from build123d import *

# Parameters (mm, degrees)
ESQUISSE1_R                  = 32.75
ESQUISSE1_R_2                = 30.75
BOSS_EXTRU_1_DEPTH           = 25
ESQUISSE2_W                  = 30
ESQUISSE2_H                  = 4
ENL_V_MAT_EXTRU_1_DEPTH      = 53.631976972
R_P_TITION_CIRCULAIRE1_COUNT = 4


with BuildPart() as part:
    # Esquisse1 → Boss.-Extru.1 (new body)
    with BuildSketch(Plane(origin=(0, 0, 0), x_dir=(1, 0, 0), z_dir=(0, 1, 0))):
        with Locations(Location((0, 0, 0), (0, 0, 270))):
            Circle(ESQUISSE1_R)
        with Locations(Location((0, 0, 0), (0, 0, 270))):
            Circle(ESQUISSE1_R_2, mode=Mode.SUBTRACT)
    extrude(amount=BOSS_EXTRU_1_DEPTH)

    # Esquisse2 → Enlèv. mat.-Extru.1 (cut, through all)
    with BuildSketch(Plane.XY):
        with Locations((0, 17)):
            Rectangle(ESQUISSE2_W, ESQUISSE2_H)
    enl_v_mat_extru_1 = extrude(amount=-ENL_V_MAT_EXTRU_1_DEPTH, mode=Mode.SUBTRACT)

    # Répétition circulaire1: Enlèv. mat.-Extru.1 ×4 about axis
    r_p_tition_circulaire1_axis = Axis((0, 0, 0), (0, 1, 0))
    for i in range(1, R_P_TITION_CIRCULAIRE1_COUNT):
        add(enl_v_mat_extru_1.rotate(r_p_tition_circulaire1_axis, i * 360 / R_P_TITION_CIRCULAIRE1_COUNT), mode=Mode.SUBTRACT)


solid = part.part
Geometry: final body of the model. Coordinates: model frame, mm. A direction names the side the tool comes from. Give positions to 0.01 mm unless a question says otherwise; leave off trailing zeros. Loops run counter-clockwise (first coordinate to the right, second up) from the corner with the lowest first, then second, coordinate; pieces in that order, holes last. Notation, with made-up numbers: M 45,89.25 L 95,89.25 A31 ccw 95,128.25 Z; hole C 3.25,-3.5 d1. An arc over 180 degrees is marked long. Put each result on its own line as item: value. Start each with the question number.
1) Cut plane A-A (z = 0). Output: boundary loops of the cut face in (x, y).
2) Contact query for flat-ended pins moving along their axis: pin 1 (6 mm diameter, centred on y = 7, z = 10, fed in from +X); pin 2 (1.8 mm diameter, centred on x = -28, y = 17.5, fed in from +Z); pin 3 (1.8 mm diameter, centred on y = 18, z = 28.5, fed in from -X). Output: stop coordinate, or through.
3) Cut plane B-B (x = 0). Output: boundary loops of the cut face in (y, z), then the cut area to 3 significant figures.
4) Ray query, line 1 along X through (y, z) = (19.75, 0); line 2 along Y through (x, z) = (29, 14.5); line 3 along X through (y, z) = (8.75, -15). Return the intervals inside material, ascending.
5) Cut plane C-C (y = 11.5). Output: boundary loops of the cut face in (x, z), then the cut area to 3 significant figures.
6) Pull-direction query (X, two-part tool) for faces 1 (the flat face through (31, 15, 0)), 2 (the flat face through (-15, 17, 28)); classes: pulls with the +X half, pulls with the -X half, needs draft (parallel to the pull), parting line crosses it, or undercut.
7) Access query for faces 3 (the flat face through (-31, 19, 0)), 4 (the flat face through (0, 15, 31)), 5 (the flat face through (9.9, 0, -29.3)). Directions: +Z, -Z, +X, -X, +Y, -Y. A direction counts if a zero-diameter tool reaches every point of the face in a straight line with its end or side. Return the directions, or none.
8) Cut plane D-D (x = -26). Output: boundary loops of the cut face in (y, z), then the cut area to 3 significant figures.
Verdict:
1. outline: M -32.75,0 L -30.75,0 L -30.75,15 L -32.75,15 Z; M -32.75,19 L -30.75,19 L -30.75,25 L -32.75,25 Z; M 30.75,0 L 32.75,0 L 32.75,15 L 30.75,15 Z; M 30.75,19 L 32.75,19 L 32.75,25 L 30.75,25 Z
2. pin 1: x = 31.99
2. pin 2: z = 18.39
2. pin 3: x = -17.63
3. outline: M 0,-32.75 L 15,-32.75 L 15,-30.75 L 0,-30.75 Z; M 0,30.75 L 15,30.75 L 15,32.75 L 0,32.75 Z; M 19,-32.75 L 25,-32.75 L 25,-30.75 L 19,-30.75 Z; M 19,30.75 L 25,30.75 L 25,32.75 L 19,32.75 Z
3. area: 84.0 mm2
4. line 1: -32.75 to -30.75, 30.75 to 32.75
4. line 2: 0 to 15, 19 to 25
4. line 3: -29.11 to -26.84, 26.84 to 29.11
5. outline: C 0,0 d65.5; hole C 0,0 d61.5
5. area: 399 mm2
6. face 1: needs draft
6. face 2: undercut
7. face 3: +X, -X
7. face 4: +Z, -Z
7. face 5: +Z, -Z, +X, -X, -Y
8. outline: M 0,-19.91 L 25,-19.91 L 25,-16.42 L 0,-16.42 Z; M 0,16.42 L 25,16.42 L 25,19.91 L 0,19.91 Z
8. area: 175 mm2
